Could you check a few things on this drawing? It's one solid part, dimensions in mm from its lowest x, y, z. Give positions to 0.01 mm unless a question says otherwise; leave off trailing zeros. Write each loop counter-clockwise with the first axis right and the second up, starting at its lowest first coordinate (ties: lowest second). Pieces come first, ordered by that corner, then holes. Notation, with made-up numbers: M 67,-34 L 110,-34 A20 cw 110,-27 Z; hole C 12,9 d1. An arc over 180 degrees is marked long. Answer as CSV lines item,"result". Start each with the question number.
Q1. Suppose I cut it at C-C (x = 38.1). Write out the boundary of the cut face in (y, z).
Q2. Suppose I cut it at B-B (y = 2.25). Write out the boundary of the cut face in (x, z) (1 decimal), then the cut area to 3 significant figures.
Q3. Suppose I cut it at A-A (z = 38.1). Write out the boundary of the cut face in (x, y), then the cut area to 3 significant figures.
Q4. Suppose I cut it at D-D (z = 61). Count the separate pieces of the cut face and the enclosed holes in it, then the cut area to 3 significant figures.
Q5. If I drill on line 1 along X through (y, z) = (3, 52) (1 decimal); line 2 along Z through (x, y) = (27, 2.25); line 3 along Z through (x, y) = (14, 3), over which ranges is the centre line in solid material (lowest first)?
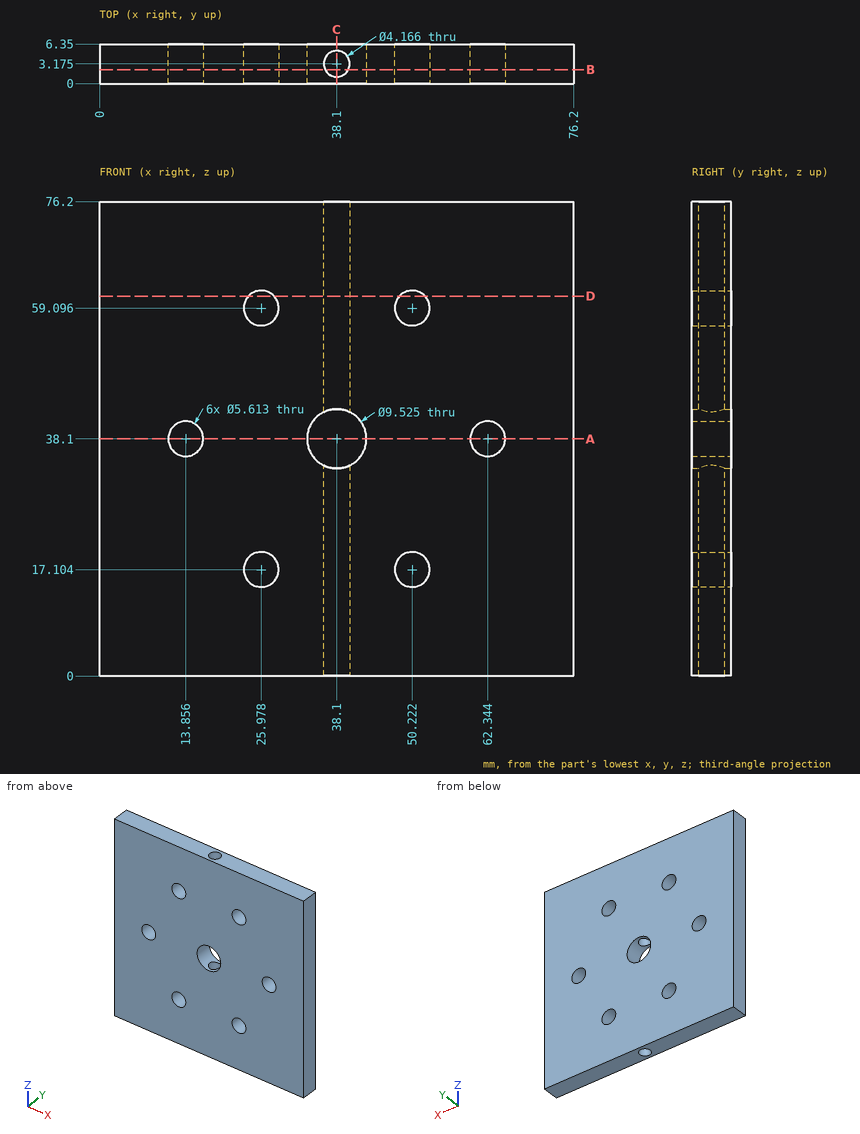
Resolved:
1,outline,"M 0,0 L 1.09,0 L 1.09,33.34 L 0,33.34 Z; M 0,42.86 L 1.09,42.86 L 1.09,76.2 L 0,76.2 Z; M 5.26,0 L 6.35,0 L 6.35,33.34 L 5.26,33.34 Z; M 5.26,42.86 L 6.35,42.86 L 6.35,76.2 L 5.26,76.2 Z"
2,outline,"M 0,0 L 36.2,0 L 36.2,33.7 A4.8 cw 36.2,42.5 L 36.2,76.2 L 0,76.2 Z; M 40,0 L 76.2,0 L 76.2,76.2 L 40,76.2 L 40,42.5 A4.8 cw 40,33.7 Z; hole C 13.9,38.1 d5.6; hole C 26,17.1 d5.6; hole C 26,59.1 d5.6; hole C 50.2,17.1 d5.6; hole C 50.2,59.1 d5.6; hole C 62.3,38.1 d5.6"
2,area,"5,340 mm^2"
3,outline,"M 0,0 L 11.05,0 L 11.05,6.35 L 0,6.35 Z; M 16.66,0 L 33.34,0 L 33.34,6.35 L 16.66,6.35 Z; M 42.86,0 L 59.54,0 L 59.54,6.35 L 42.86,6.35 Z; M 65.15,0 L 76.2,0 L 76.2,6.35 L 65.15,6.35 Z"
3,area,"352 mm^2"
4,separate pieces,"3"
4,enclosed holes,"1"
4,area,"418 mm^2"
5,line 1,"0 to 36, 40.2 to 76.2"
5,line 2,"0 to 14.49, 19.72 to 56.48, 61.71 to 76.2"
5,line 3,"0 to 35.3, 40.9 to 76.2"
